Autodesk Inventor part; units mm, degrees
ref_plane "YZ Plane" through (0, 0, 0) normal (1, 0, 0) x (0, 1, 0)
ref_plane "XZ Plane" through (0, 0, 0) normal (0, 1, 0) x (-1, 0, 0)
ref_plane "XY Plane" through (0, 0, 0) normal (0, 0, 1) x (1, 0, 0)
sketch "草图1" plane through (0, 0, 0) normal (1, 0, 0) x (0, 1, 0)
  line L0 (-12.5, 21) -> (12.5, 21)
  line L1 (12.5, 21) -> (12.5, -21)
  line L2 (12.5, -21) -> (-12.5, -21)
  line L3 (-12.5, -21) -> (-12.5, 21)
  line L4 (-12.5, 21) -> (12.5, -21) construction
  line L5 (12.5, 21) -> (-12.5, -21) construction
  line L6 (-7.5, -15) -> (4.5, -15) construction
  line L7 (4.5, -15) -> (4.5, 15) construction
  line L8 (4.5, 15) -> (-7.5, 15) construction
  line L9 (-7.5, 15) -> (-7.5, -15) construction
  line L10 (-7.5, -15) -> (4.5, 15) construction
  line L11 (4.5, -15) -> (-7.5, 15) construction
  line L12 (18.2853, 0) -> (0, 0) construction
  circle A0 centre (4.5, -15) radius 1.75
  circle A1 centre (4.5, 15) radius 1.75
  circle A2 centre (-7.5, 15) radius 1.75
  circle A3 centre (-7.5, 0) radius 1.75
  circle A4 centre (-7.5, -15) radius 1.75
  point P0 (-1.5, 0)
  dimension "d0" = 42
  dimension "d1" = 25
  dimension "d4" = 8
  dimension "d5" = 20
  dimension "d6" = 30
  dimension "d7" = 3.5
  dimension "d8" = 3.5
  dimension "d9" = 3.5
  dimension "d10" = 3.5
  dimension "d11" = 3.5
extrude "拉伸1" add sketch "草图1" along normal blind 4
fillet "圆角1" radius 3 2 edges at (2, -12.5, -21) (2, -12.5, 21)
sketch "草图2" plane through (4, 0, 0) normal (1, 0, 0) x (0, 0, -1)
  line L0 (21, 12.5) -> (-21, 12.5)
  line L1 (9, -1.5) -> (-9, -1.5)
  line L2 (-9, -1.5) -> (-9, 12.5)
  line L3 (-9, 12.5) -> (9, 12.5)
  line L4 (9, 12.5) -> (9, -1.5)
  line L5 (9, -1.5) -> (-9, 12.5) construction
  line L6 (-9, -1.5) -> (9, 12.5) construction
  line L7 (0, -21.7484) -> (0, 21.3342) construction
  point P0 (0, 0)
  point P1 (0, 5.5)
  point P2 (9, 12.5)
  dimension "d15" = 18
  dimension "d16" = 14
extrude "拉伸2" add sketch "草图2" along normal blind 114
sketch "草图3" plane through (118, 0, 0) normal (1, 0, 0) x (0, 0, -1)
  arc A0 (-21, -9.5) -> (-18, -12.5) centre (-18, -9.5) ccw
  line L0 (-21, 12.5) -> (-21, -9.5)
  line L1 (21, 12.5) -> (-21, 12.5)
  line L2 (21, -9.5) -> (21, 12.5)
  arc A1 (18, -12.5) -> (21, -9.5) centre (18, -9.5) ccw
  line L3 (-18, -12.5) -> (18, -12.5)
  circle A2 centre (15, -7.5) radius 1.75
  circle A3 centre (0, -7.5) radius 1.75
  circle A4 centre (-15, -7.5) radius 1.75
  circle A5 centre (-15, 4.5) radius 1.75
  circle A6 centre (15, 4.5) radius 1.75
  point P0 (0, 0)
extrude "拉伸3" add sketch "草图3" along normal blind 4
chamfer "倒角1" distance 2 angle 45 2 edges at (61, -1.5, -9) (61, -1.5, 9)
sketch "草图4" plane through (0, 12.5, 21) normal (0, 1, 0) x (1, 0, 0)
  line L0 (61, 0.1174) -> (61, 41.8826) construction
  line L1 (122, 42) -> (122, 0)
  line L2 (0, 42) -> (0, 0)
  circle A0 centre (61, 21) radius 2.1
  line L3 (122, 21) -> (0, 21) construction
  circle A1 centre (46, 21) radius 2.1
  circle A2 centre (31, 21) radius 2.1
  circle A3 centre (16, 21) radius 2.1
  circle A4 centre (76, 21) radius 2.1
  circle A5 centre (61, 21) radius 2.1
  circle A6 centre (46, 21) radius 2.1
  circle A7 centre (31, 21) radius 2.1
  circle A8 centre (91, 21) radius 2.1
  circle A9 centre (76, 21) radius 2.1
  circle A10 centre (61, 21) radius 2.1
  circle A11 centre (46, 21) radius 2.1
  circle A12 centre (106, 21) radius 2.1
  circle A13 centre (91, 21) radius 2.1
  circle A14 centre (76, 21) radius 2.1
  circle A15 centre (61, 21) radius 2.1
  dimension "d24" = 61
  dimension "d25" = 61
  dimension "d26" = 4.2
  dimension "d29" = 15
  dimension "d32" = 15
extrude "拉伸4" cut sketch "草图4" against normal through all
properties part number "加强梁"
The listing builds one solid part. Answer for the finished solid, in the listing's coordinates (mm). A direction names the side the tool comes from. Coordinates: 2 decimals unless noted, no trailing zeros. Order: outer loops, then holes, each group sorted by start corner. A loop starts at its lowest first (then second) coordinate and runs counter-clockwise, first axis right, second up. Notation, with made-up numbers: (89, 22) -> (106, 22) arc R16 ccw to (106, 30) -> close; hole circle Ø6 at (47.25, 51). An arc over 180 degrees is marked (long way). Answer in a Markdown table with one row per item. Add a question column.
Item 1: Find section B-B (z = 12). Write down the section's boundary in (x, y), then the cut area to 3 significant figures.
Item 2: Which of the six approach directions +Z, -Z, +X, -X, +Y, -Y give full straight-line access (tool end or side, diameter ignored) to faces 1 (the face through (61.8, -0.5, 8)), 2 (the face through (60, 7, -9)), 3 (the face through (118, -3, 0)), 4 (the face through (60, -1.5, -3)), 5 (the face through (1.972, 4.272, -16.735))?
Item 3: Find section C-C (y = 4.5). State how many separate pieces and enclosed holes the cut face has, then the cut area to 3 significant figures.
Item 4: Find the intervals of material crossed by L1, parallel to Z at x = 2.2, y = -7.5; L2, parallel to X at y = -8.25, z = -13; L3, parallel to Z at x = 91, y = 0.5, in increasing order. Write a range as from..to.
Item 5: Find section A-A (x = 46). Write down the section's boundary in (y, z), then the cut area to 3 significant figures.
Item 6: Each of these flat-tipped pins is pushed along its axis until it touches: P1, Ø8, axis at x = 39, y = 2.5, coming from the -Z side; P2, Ø5, axis at x = 61, z = 0, coming from the +Y side; P3, Ø12, axis at x = 97, z = 7.5, coming from the -Y side; P4, Ø3, axis at x = 17, y = 6.5, coming from the +Z side. Where does it stop, or does it pass through?
Item 7: Determine the mould class of faces 6 (the face through (122, 0, 0)), 7 (the face through (2.03, -11.64, -20.1)), 8 (the face through (62.94, 5.6, 0.8)) for opening direction X: +X half, -X half, draft (parallel to the pull), parting line (faces both ways), or undercut.
Item 8: Find section D-D (x = 111.5). Write down the section's boundary in (y, z).
Result set:
| question | item | result |
|---|---|---|
| 1 | outline | (0, -12.5) -> (4, -12.5) -> (4, 12.5) -> (0, 12.5) -> close; (118, -12.5) -> (122, -12.5) -> (122, 12.5) -> (118, 12.5) -> close |
| 1 | area | 200 mm² |
| 2 | face 1 | +Z, -Y |
| 2 | face 2 | -Z, +Y, -Y |
| 2 | face 3 | -Y |
| 2 | face 4 | +Z, -Z, -Y |
| 2 | face 5 | +X, -X |
| 3 | separate pieces | 5 |
| 3 | enclosed holes | 7 |
| 3 | area | 2,240 mm² |
| 4 | L1 | z = -21..-16.75, -13.25..-1.75, 1.75..13.25, 16.75..21 |
| 4 | L2 | x = 0..4, 118..122 |
| 4 | L3 | z = -9..-2.1, 2.1..9 |
| 5 | outline | (-1.5, -7) -> (0.5, -9) -> (12.5, -9) -> (12.5, -2.1) -> (-1.5, -2.1) -> close; (-1.5, 2.1) -> (12.5, 2.1) -> (12.5, 9) -> (0.5, 9) -> (-1.5, 7) -> close |
| 5 | area | 189 mm² |
| 6 | P1 | stops at z = -9 |
| 6 | P2 | stops at y = 12.5 |
| 6 | P3 | stops at y = -1.5 |
| 6 | P4 | stops at z = 9 |
| 7 | face 6 | +X half |
| 7 | face 7 | draft |
| 7 | face 8 | undercut |
| 8 | outline | (-1.5, -7) -> (0.5, -9) -> (12.5, -9) -> (12.5, 9) -> (0.5, 9) -> (-1.5, 7) -> close |
